For this review, take the finished solid that the model builds, in its own axes (mm). Face numbers are marked on the shaded views. Coordinates: 2 decimals unless noted, no trailing zeros. Loops run counter-clockwise (first coordinate to the right, second up) from the corner with the lowest first, then second, coordinate; pieces in that order, holes last. Notation, with made-up numbers: (9, 60.25) - (67, 60.25) arc R24 cw to (67, 94.25) - close; hole circle Ø11 at (6.5, -16). An arc over 180 degrees is marked (long way). Answer as a JSON object with one key per item and string values. Group by question number.
Item 1: We need section A-A (y = -28.5). Give the boundary of the cut face in (x, z) (3 decimals), then the cut area to 3 significant figures.
Item 2: Clearance check with flat-ended pins moving along their axes: pin 1 (0.6 mm diameter, centred on x = 22, y = -71, fed in from +Z); pin 2 (12 mm diameter, centred on x = -30.5, y = -62, fed in from +Z); pin 3 (10 mm diameter, centred on x = -4.5, y = -130, fed in from +Z). State where each tip first meets the part, or that it passes through.
Item 3: We need section C-C (x = -16). Give the boundary of the cut face in (y, z), then the cut area to 3 significant figures.
Item 4: We need section D-D (x = 29.5). Give the boundary of the cut face in (y, z), then the cut area to 3 significant figures.
Item 5: To check wall thickness, follow line 1 (Z direction, x = 6, y = -139); line 2 (X direction, y = -84, z = 3.5); line 3 (X direction, y = -33, z = 9). State the ranges of each line that lie inside material, in increasing order.
Item 6: We need section B-B (z = 19). Give the boundary of the cut face in (x, y), then the cut area to 3 significant figures.
Item 7: Mouldability with a two-part tool opening along X and no side actions: class the marked faces 1, 2, 3 and 4 as released by +X, released by -X, zero draft, split by the parting line, or undercut.
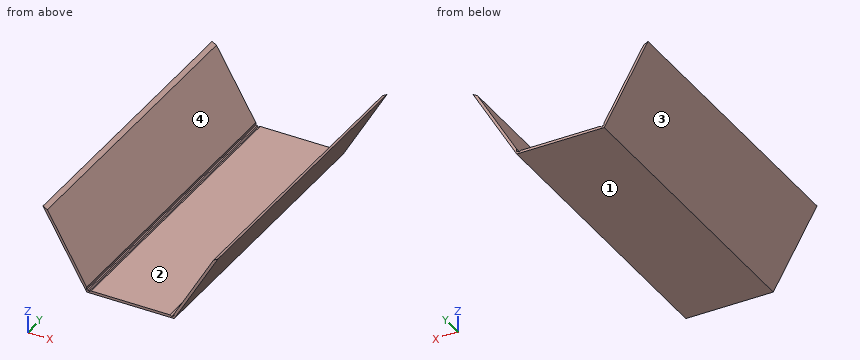
from build123d import *

# Parameters (mm, degrees)
F1_DEPTH = 152.4
F2_DEPTH = 74.93
F3_DEPTH = 74.93
F4_DEPTH = 74.93


with BuildPart() as f1:
    # F0 (on Front) → F1 (new body)
    with BuildSketch(Plane.XZ):
        Polygon((43.9940905122, 38.1), (21.9970452561, 76.2), (-21.9970452561, 76.2), (-43.9940905122, 38.1), (-21.9970452561, 0), (21.9970452561, 0), align=None)
    extrude(amount=F1_DEPTH)

    # F2 (cut): a face of the model
    f2_faces = [f1.faces().sort_by_distance(p)[0] for p in [
        (32.9955678842, -76.2, 57.15),
    ]]
    extrude(f2_faces, amount=-F2_DEPTH, mode=Mode.SUBTRACT)

    # F3 (cut): a face of the model
    f3_faces = [f1.faces().sort_by_distance(p)[0] for p in [
        (0, -76.2, 76.2),
    ]]
    extrude(f3_faces, amount=-F3_DEPTH, mode=Mode.SUBTRACT)

    # F4 (cut): a face of the model
    f4_faces = [f1.faces().sort_by_distance(p)[0] for p in [
        (-32.9955678842, -76.2, 57.15),
    ]]
    extrude(f4_faces, amount=-F4_DEPTH, mode=Mode.SUBTRACT)


solid = f1.part
Check sheet entries:
{
 "1": {"outline": "(-43.994, 38.1) - (-21.997, 0) - (21.997, 0) - (43.994, 38.1) - (41.794, 36.83) - (21.997, 2.54) - (21.997, 1.27) - (21.264, 1.27) - (20.897, 0.635) - (19.797, 1.27) - (-19.797, 1.27) - (-20.897, 0.635) - (-21.264, 1.27) - (-21.997, 1.27) - (-21.997, 2.54) - (-41.794, 36.83) - close", "area": "161 mm2"},
 "2": {"pin 1": "stops at z = 3.06", "pin 2": "stops at z = 27.66", "pin 3": "stops at z = 1.27"},
 "3": {"outline": "(-152.4, 0) - (0, 0) - (0, 1.27) - (-152.4, 1.27) - close", "area": "194 mm2"},
 "4": {"outline": "(-152.4, 13) - (0, 13) - (0, 15.54) - (-152.4, 15.54) - close", "area": "387 mm2"},
 "5": {"line 1": "z = 0 to 1.27", "line 2": "x = -24.02 to -22.55, 22.55 to 24.02", "line 3": "x = -27.19 to -25.73, 25.73 to 27.19"},
 "6": {"outline": "(-32.97, -152.4) - (-31.5, -152.4) - (-31.5, 0) - (-32.97, 0) - close; (31.5, -152.4) - (32.97, -152.4) - (32.97, 0) - (31.5, 0) - close", "area": "447 mm2"},
 "7": {"face 1": "zero draft", "face 2": "undercut", "face 3": "released by -X", "face 4": "undercut"}
}
